Geometry check sheet. Reference: the model listing, model coordinates, mm. Round coordinates to 2 decimals unless told otherwise and drop trailing zeros. Order: outer loops, then holes, each group sorted by start corner. A loop starts at its lowest first (then second) coordinate and runs counter-clockwise, first axis right, second up. Notation, with made-up numbers: M 36.5,36 L 87.5,36 A19 cw 87.5,63 Z; hole C 24.5,33.25 d7. An arc over 180 degrees is marked long. Answer as a JSON object with one key per item and string values. Group by question number.
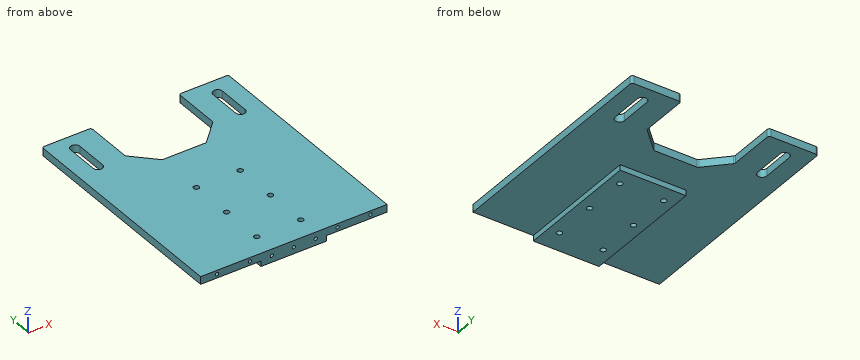
```python
from build123d import *

# Parameters (mm, degrees)
SKETCH1_R           = 2.5
BOSS_EXTRUDE1_DEPTH = 12
CUT_EXTRUDE1_DEPTH  = 5
FILLET1_R           = 2
SKETCH4_R           = 1.5
CUT_EXTRUDE2_DEPTH  = 5


with BuildPart() as part:
    # Sketch1 → Boss-Extrude1 (new body)
    with BuildSketch(Plane.XY):
        Polygon((0, 210), (45, 210), (45, 165), (65, 145), (105, 145), (125, 165), (125, 210), (170, 210), (170, 0), (0, 0), align=None)
        with Locations((65, 20)):
            Circle(SKETCH1_R, mode=Mode.SUBTRACT)
        with Locations((65, 60)):
            Circle(SKETCH1_R, mode=Mode.SUBTRACT)
        with Locations((65, 100)):
            Circle(SKETCH1_R, mode=Mode.SUBTRACT)
        with Locations(Location((105, 100, 0), (0, 0, 180))):
            Circle(SKETCH1_R, mode=Mode.SUBTRACT)
        with Locations(Location((105, 60, 0), (0, 0, 180))):
            Circle(SKETCH1_R, mode=Mode.SUBTRACT)
        with Locations(Location((105, 20, 0), (0, 0, 180))):
            Circle(SKETCH1_R, mode=Mode.SUBTRACT)
        with BuildLine():
            Line((154.25, 195), (154.25, 165))
            ThreePointArc((154.25, 165), (150, 160.75), (145.75, 165))
            Line((145.75, 165), (145.75, 195))
            ThreePointArc((145.75, 195), (150, 199.25), (154.25, 195))
        make_face(mode=Mode.SUBTRACT)
        with BuildLine():
            Line((15.75, 195), (15.75, 165))
            ThreePointArc((15.75, 165), (20, 160.75), (24.25, 165))
            Line((24.25, 165), (24.25, 195))
            ThreePointArc((24.25, 195), (20, 199.25), (15.75, 195))
        make_face(mode=Mode.SUBTRACT)
    extrude(amount=BOSS_EXTRUDE1_DEPTH)

    # Sketch3 → Cut-Extrude1 (cut)
    with BuildSketch(Plane(origin=(0, 0, 0), x_dir=(-1, 0, 0), z_dir=(0, 0, -1))):
        Polygon((0, 0), (-55, 0), (-55, 115), (-115, 115), (-115, 0), (-170, 0), (-170, 210), (-115, 210), (-55, 210), (0, 210), align=None)
    extrude(amount=-CUT_EXTRUDE1_DEPTH, mode=Mode.SUBTRACT)

    # Fillet1
    fillet1_edges = [part.edges().sort_by_distance(p)[0] for p in [
        (0, 210, 8.5),
        (45, 210, 8.5),
        (45, 165, 8.5),
        (65, 145, 8.5),
        (105, 145, 8.5),
        (125, 165, 8.5),
        (125, 210, 8.5),
        (170, 210, 8.5),
    ]]
    fillet(fillet1_edges, radius=FILLET1_R)

    # Sketch4 → Cut-Extrude2 (cut)
    with BuildSketch(Plane.XZ):
        with Locations((85, 6)):
            Circle(SKETCH4_R)
        with Locations((105, 6)):
            Circle(SKETCH4_R)
        with Locations((155, 8.5)):
            Circle(SKETCH4_R)
        with Locations((125, 8.5)):
            Circle(SKETCH4_R)
        with Locations(Location((15, 8.5, 0), (0, 0, 180))):
            Circle(SKETCH4_R)
        with Locations(Location((45, 8.5, 0), (0, 0, 180))):
            Circle(SKETCH4_R)
        with Locations(Location((65, 6, 0), (0, 0, 180))):
            Circle(SKETCH4_R)
    extrude(amount=-CUT_EXTRUDE2_DEPTH, mode=Mode.SUBTRACT)


solid = part.part
```
1) Thickness scan on line 1 along Y through (x, z) = (65.5, 9); line 2 along Y through (x, z) = (65, 4); line 3 along Z through (x, y) = (155, 2.2). Record the ranges inside material, lowest first. Write a range as [from, to].
2) Sectioned sample at A-A (y = 60). Record the boundary of the cut face in (x, z), then the cut area to 3 significant figures.
3) Sectioned sample at B-B (x = 20). Record the boundary of the cut face in (y, z).
4) Go/stop test with flat-tipped pins: P1, Ø1, axis at x = 93.5, z = 1.5, coming from the +Y side; P2, Ø0.9, axis at x = 125.5, z = 9, coming from the -Y side; P3, Ø3, axis at x = 105, y = 100, coming from the -Z side; P4, Ø5.5, axis at x = 90, z = 7, coming from the +Y side. Record where each tip stops, or that it passes through.
5) Sectioned sample at C-C (y = 136). Record the boundary of the cut face in (x, z).
Final values:
{
 "1": {"line 1": "y = [0, 17.55], [22.45, 57.55], [62.45, 97.55], [102.45, 145.03]", "line 2": "y = [0, 17.5], [22.5, 57.5], [62.5, 97.5], [102.5, 115]", "line 3": "z = [5, 7], [10, 12]"},
 "2": {"outline": "M 0,5 L 55,5 L 55,0 L 62.5,0 L 62.5,12 L 0,12 Z; M 67.5,0 L 102.5,0 L 102.5,12 L 67.5,12 Z; M 107.5,0 L 115,0 L 115,5 L 170,5 L 170,12 L 107.5,12 Z", "area": "1,370 mm^2"},
 "3": {"outline": "M 0,5 L 160.75,5 L 160.75,12 L 0,12 Z; M 199.25,5 L 210,5 L 210,12 L 199.25,12 Z"},
 "4": {"P1": "stops at y = 115", "P2": "stops at y = 5", "P3": "passes through", "P4": "stops at y = 145"},
 "5": {"outline": "M 0,5 L 170,5 L 170,12 L 0,12 Z"}
}
